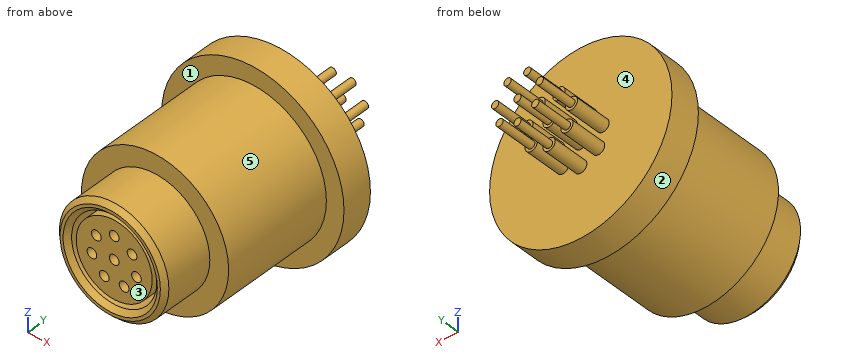
```python
from build123d import *

# Parameters (mm, degrees)
SKETCH1_R            = 4.5
SKETCH1_R_2          = 3.5
BOSS_EXTRUDE1_DEPTH  = 4.25
SKETCH2_R            = 4.25
BOSS_EXTRUDE2_DEPTH  = 1.3
SKETCH3_R            = 6.05
BOSS_EXTRUDE3_DEPTH  = 9.25
SKETCH6_R            = 7.5
BOSS_EXTRUDE5_DEPTH  = 2.5
SKETCH10_R           = 0.5
BOSS_EXTRUDE7_DEPTH  = 3
SKETCH11_R           = 0.3
BOSS_EXTRUDE8_DEPTH  = 3
SKETCH11_3_R         = 0.3
BOSS_EXTRUDE9_DEPTH  = 3
CHAMFER1_SIZE        = 0.375
CHAMFER2_SIZE        = 0.375
BOSS_EXTRUDE12_REACH = 24.375
BOSS_EXTRUDE12_START = -0.375
SKETCH19_R           = 3.125
SKETCH20_R           = 0.4
CUT_EXTRUDE3_DEPTH   = 3.875


with BuildPart() as part:
    # Sketch1 → Boss-Extrude1 (new body)
    with BuildSketch(Plane(origin=(0, 0, 0), x_dir=(1, 0, 0), z_dir=(0, 1, 0))):
        Circle(SKETCH1_R)
        Circle(SKETCH1_R_2, mode=Mode.SUBTRACT)
    extrude(amount=BOSS_EXTRUDE1_DEPTH)

    # Sketch2 → Boss-Extrude2 (add)
    with BuildSketch(Plane(origin=(0, 4.25, 0), x_dir=(1, 0, 0), z_dir=(0, 1, 0))):
        Circle(SKETCH2_R)
    extrude(amount=-BOSS_EXTRUDE2_DEPTH)

    # Sketch3 → Boss-Extrude3 (add)
    with BuildSketch(Plane(origin=(0, 4.25, 0), x_dir=(1, 0, 0), z_dir=(0, 1, 0))):
        Circle(SKETCH3_R)
    extrude(amount=BOSS_EXTRUDE3_DEPTH)

    # Sketch6 → Boss-Extrude5 (add)
    with BuildSketch(Plane(origin=(0, 13.5, 0), x_dir=(1, 0, 0), z_dir=(0, 1, 0))):
        Circle(SKETCH6_R)
    extrude(amount=BOSS_EXTRUDE5_DEPTH)

    # Sketch10 → Boss-Extrude7 (add)
    with BuildSketch(Plane(origin=(0, 16, 0), x_dir=(1, 0, 0), z_dir=(0, 1, 0))):
        Circle(SKETCH10_R)
        with Locations((0, 1.88)):
            Circle(SKETCH10_R)
        with Locations((1.469843187, 1.172160827)):
            Circle(SKETCH10_R)
        with Locations((1.832864475, -0.418339356)):
            Circle(SKETCH10_R)
        with Locations((0.81570143, -1.693821472)):
            Circle(SKETCH10_R)
        with Locations((-0.81570143, -1.693821472)):
            Circle(SKETCH10_R)
        with Locations((-1.832864475, -0.418339356)):
            Circle(SKETCH10_R)
        with Locations((-1.469843187, 1.172160827)):
            Circle(SKETCH10_R)
    extrude(amount=BOSS_EXTRUDE7_DEPTH)

    # Sketch11 → Boss-Extrude8 (add)
    with BuildSketch(Plane(origin=(0, 19, 0), x_dir=(1, 0, 0), z_dir=(0, 1, 0))):
        with Locations((-0.81570143, -1.693821472)):
            Circle(SKETCH11_R)
    extrude(amount=BOSS_EXTRUDE8_DEPTH)

    # Sketch11<3> → Boss-Extrude9 (add)
    with BuildSketch(Plane(origin=(0, 19, 0), x_dir=(1, 0, 0), z_dir=(0, 1, 0))):
        Circle(SKETCH11_3_R)
        with Locations((0, 1.88)):
            Circle(SKETCH11_3_R)
        with Locations((1.469843187, 1.172160827)):
            Circle(SKETCH11_3_R)
        with Locations((1.832864475, -0.418339356)):
            Circle(SKETCH11_3_R)
        with Locations((0.81570143, -1.693821472)):
            Circle(SKETCH11_3_R)
        with Locations((-0.81570143, -1.693821472)):
            Circle(SKETCH11_3_R)
        with Locations((-1.832864475, -0.418339356)):
            Circle(SKETCH11_3_R)
        with Locations((-1.469843187, 1.172160827)):
            Circle(SKETCH11_3_R)
    extrude(amount=BOSS_EXTRUDE9_DEPTH)

    # Chamfer1
    chamfer1_edges = [part.edges().sort_by_distance(p)[0] for p in [
        (-4.5, 0, 0),
    ]]
    chamfer(chamfer1_edges, length=CHAMFER1_SIZE)

    # Chamfer2
    chamfer2_edges = [part.edges().sort_by_distance(p)[0] for p in [
        (-3.5, 2.95, 0),
        (-3.5, 0, 0),
    ]]
    chamfer(chamfer2_edges, length=CHAMFER2_SIZE)

    # Sketch19 → Boss-Extrude12 (add, up to next)
    with BuildSketch(Plane.XZ.offset(BOSS_EXTRUDE12_START), mode=Mode.PRIVATE) as boss_extrude12_sk1:
        Circle(SKETCH19_R)
    boss_extrude12_tool1 = extrude(boss_extrude12_sk1.sketch, amount=-BOSS_EXTRUDE12_REACH, mode=Mode.PRIVATE) - part.part
    add(boss_extrude12_tool1.solids().sort_by_distance((0, 0.375, 0))[0])

    # Sketch20 → Cut-Extrude3 (cut)
    with BuildSketch(Plane.XZ.offset(-0.375)):
        Circle(SKETCH20_R)
        with Locations((0, 1.88)):
            Circle(SKETCH20_R)
        with Locations((1.469843187, 1.172160827)):
            Circle(SKETCH20_R)
        with Locations((1.832864475, -0.418339356)):
            Circle(SKETCH20_R)
        with Locations((0.81570143, -1.693821472)):
            Circle(SKETCH20_R)
        with Locations((-0.81570143, -1.693821472)):
            Circle(SKETCH20_R)
        with Locations((-1.832864475, -0.418339356)):
            Circle(SKETCH20_R)
        with Locations((-1.469843187, 1.172160827)):
            Circle(SKETCH20_R)
    extrude(amount=-CUT_EXTRUDE3_DEPTH, mode=Mode.SUBTRACT)


solid = part.part
```
Work out the finished part from the listing and answer in its coordinate system (mm). Face numbers are marked on the shaded views. A direction names the side the tool comes from. Give positions to 0.01 mm unless a question says otherwise; leave off trailing zeros. Write each loop counter-clockwise with the first axis right and the second up, starting at its lowest first coordinate (ties: lowest second). Pieces come first, ordered by that corner, then holes. Notation, with made-up numbers: (30, 70) -> (48, 70) arc R11 cw to (48, 84) -> close; hole circle Ø10 at (78, 14.25). An arc over 180 degrees is marked (long way). Write item = value, one per line.
Q1. Section D-D on y = 17.5 is taken. Determine the outline of the cut face in (x, z), and give its area (3 significant figures).
Computed values:
outline = circle Ø1 at (-1.83, 0.42); circle Ø1 at (-1.47, -1.17); circle Ø1 at (-0.82, 1.69); circle Ø1 at (0, -1.88); circle Ø1 at (0, 0); circle Ø1 at (0.82, 1.69); circle Ø1 at (1.47, -1.17); circle Ø1 at (1.83, 0.42)
area = 6.28 mm^2
Q2. A tool of negligible diameter and unlimited length cuts with its end or side. For the marked faces 4 and 5, from which of +Z, -Z, +X, -X, +Y, -Y can it reach the whole face along a straight path? Write none if from no direction.
Computed values:
face_4 = +Y
face_5 = -Y
Q3. For a pull along X with two mould halves and no side action, classify the marked faces 1, 2 and 3 as pulls with the +X half, pulls with the -X half, needs draft (parallel to the pull), parting line crosses it, or undercut.
Computed values:
face_1 = needs draft
face_2 = parting line crosses it
face_3 = undercut
Q4. Section A-A on y = 20.25 is taken. Determine the outline of the cut face in (x, z), and give its area (3 significant figures).
Computed values:
outline = circle Ø0.6 at (-1.83, 0.42); circle Ø0.6 at (-1.47, -1.17); circle Ø0.6 at (-0.82, 1.69); circle Ø0.6 at (0, -1.88); circle Ø0.6 at (0, 0); circle Ø0.6 at (0.82, 1.69); circle Ø0.6 at (1.47, -1.17); circle Ø0.6 at (1.83, 0.42)
area = 2.26 mm^2
Q5. Section B-B on z = 5 is taken. Determine the outline of the cut face in (x, y), and give its area (3 significant figures).
Computed values:
outline = (-5.59, 13.5) -> (-3.41, 13.5) -> (-3.41, 4.25) -> (3.41, 4.25) -> (3.41, 13.5) -> (5.59, 13.5) -> (5.59, 16) -> (-5.59, 16) -> close
area = 91.0 mm^2
Q6. Consider line 1 along Z through (x, y) = (0, 1.5) (3 decimals); line 2 along Z through (x, y) = (0.75, 1.5); line 3 along Y through (x, z) = (1.25, 6.75). Determine where each line is inside the solid, lowest interval first.
Computed values:
line_1 = -4.5 to -3.5, -3.125 to -0.4, 0.4 to 1.48, 2.28 to 3.125, 3.5 to 4.5
line_2 = -4.44 to -3.42, -3.03 to -2.09, -1.3 to 3.03, 3.42 to 4.44
line_3 = 13.5 to 16
Q7. Section C-C on y = 5.75 is taken. Determine the outline of the cut face in (x, z).
Computed values:
outline = circle Ø12.1 at (0, 0)
Q8. Flat-ended cylindrical pins translate along their axes: pin 1 Ø1 at (y, z) = (9, 0.5) entering from -X; pin 2 Ø0.6 at (x, z) = (-2, -0.5) entering from -Y (3 decimals); pin 3 Ø3 at (x, z) = (5.5, -3.5) entering from +Y. Find the tip coordinate at first contact, or state that the pin passes through.
Computed values:
pin_1 = -6.05
pin_2 = 0.375
pin_3 = 16
